Autodesk Fusion 360 part; units mm, degrees
sketch "Skizze1" plane through (0, 0, 0) normal (0, 1, 0) x (1, 0, 0)
  circle A0 centre (0, 0) radius 12
  circle A1 centre (0, 0) radius 15
  dimension "d1" = 24
  dimension "d2" = 30
extrude "Extrusion1" add sketch "Skizze1" along normal blind 5
extrude "Extrusion2" add sketch "Skizze1" along normal blind 10 contours A0
chamfer "Fase1" distance 2 angle 45 1 edges at (-13.9849, 0, 5.4242)
sketch "Skizze2" plane through (0, 10, 0) normal (0, 1, 0) x (-1, 0, 0)
  circle A0 centre (0, 0) radius 12
  circle A1 centre (0, 0) radius 12
  circle A2 centre (0, 0) radius 11.75
  dimension "d8" = 23.5
extrude "Extrusion3" cut sketch "Skizze2" against normal blind 5
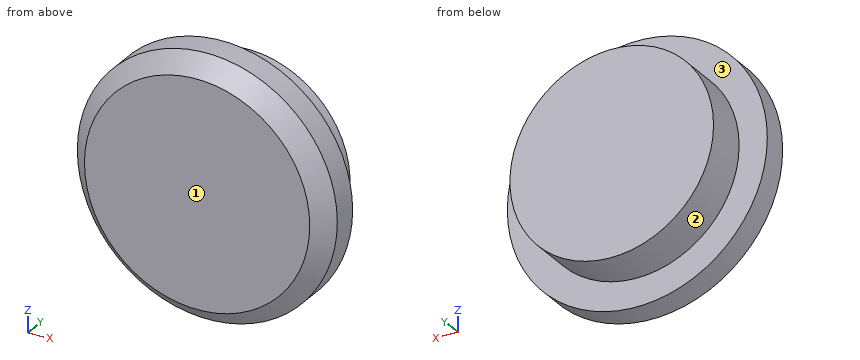
Part model, mm, in its own coordinate system. Face numbers are marked on the shaded views. Coordinates: 2 decimals unless noted, no trailing zeros. Order: outer loops, then holes, each group sorted by start corner. A loop starts at its lowest first (then second) coordinate and runs counter-clockwise, first axis right, second up. Notation, with made-up numbers: (64, 5) -> (110, 5) arc R25 ccw to (110, 27) -> close; hole circle Ø10 at (13, 21.5). An arc over 180 degrees is marked (long way). Put each result on its own line as item: value. Start each with the question number.
(1) Probe line 1 along Y through (x, z) = (10.75, -5.5); line 2 along Z through (x, y) = (-10.75, 7.75); line 3 along X through (y, z) = (4.5, 11). List the from-to ranges inside material, lowest first. Write a range as [from, to].
(2) Band-saw the part on D-D (y = 1.5). Give the cut face in (x, z).
(3) Mould opens along Y. For the marked faces 1, 2 and 3 say: pulls with the +Y half, pulls with the -Y half, needs draft (parallel to the pull), parting line crosses it, or undercut.
(4) Band-saw the part on C-C (y = 3.25). Give the cut face in (x, z), then the cut area to 3 significant figures.
(5) Band-saw the part on B-B (x = 0). Give the cut face in (y, z), then the cut area to 4 significant figures.
(6) Pin check, flat tips, straight feed: pin 1 Ø1.5 at (x, z) = (-11.5, 9.5) entering from +Y; pin 2 Ø1.5 at (y, z) = (5.5, -5.5) entering from -X; pin 3 Ø3 at (y, z) = (7.5, 12) entering from -X. Stop position of each tip, or through.
(7) Band-saw the part on A-A (z = 0). Give the cut face in (x, y), then the cut area to 4 significant figures.
Determined:
1. line 1: y = [0, 5]
1. line 2: z = [-4.74, 4.74]
1. line 3: x = [-10.2, 10.2]
2. outline: circle Ø29 at (0, 0)
3. face 1: pulls with the -Y half
3. face 2: needs draft
3. face 3: pulls with the +Y half
4. outline: circle Ø30 at (0, 0)
4. area: 707 mm²
5. outline: (0, -13) -> (2, -15) -> (5, -15) -> (5, -11.75) -> (10, -11.75) -> (10, 11.75) -> (5, 11.75) -> (5, 15) -> (2, 15) -> (0, 13) -> close
5. area: 263.5 mm²
6. pin 1: stops at y = 5
6. pin 2: stops at x = -14.16
6. pin 3: stops at x = -5.27
7. outline: (-15, 2) -> (-13, 0) -> (13, 0) -> (15, 2) -> (15, 5) -> (11.75, 5) -> (11.75, 10) -> (-11.75, 10) -> (-11.75, 5) -> (-15, 5) -> close
7. area: 263.5 mm²
